```python
from build123d import *

# Parameters (mm, degrees)
SKETCH2_R           = 25.4
BASE_CYLINDER_DEPTH = 19.05
SKETCH3_R           = 56.35625
AFT_FLANGE_DEPTH    = 9.525
BOLT_CIRCLE_D       = 2.8702
BOLT_CIRCLE_DEPTH   = 9.525


with BuildPart() as part:
    # Sketch2 → Base Cylinder (new body)
    with BuildSketch(Plane(origin=(0, 0, 0), x_dir=(1, 0, 0), z_dir=(0, 1, 0))):
        Circle(SKETCH2_R)
    extrude(amount=BASE_CYLINDER_DEPTH)

    # Sketch3 → Aft Flange (add)
    with BuildSketch(Plane.XZ):
        Circle(SKETCH3_R)
    extrude(amount=-AFT_FLANGE_DEPTH)

    # Bolt Circle
    with Locations(Plane(origin=(0, 0, 0), x_dir=(-1, 0, 0), z_dir=(0, -1, 0))):
        with Locations((-25.81275, -44.708994483), (-44.708994483, -25.81275), (-51.6255, 0), (-44.708994483, 25.81275), (-25.81275, 44.708994483), (0, 51.6255), (25.81275, 44.708994483), (44.708994483, 25.81275), (51.6255, 0), (44.708994483, -25.81275), (25.81275, -44.708994483), (0, -51.6255)):
            Hole(BOLT_CIRCLE_D / 2, depth=BOLT_CIRCLE_DEPTH)

    # Sketch17 → 3/8 NPT Tapped Hole1 (revolve, cut)
    with BuildSketch(Plane(origin=(0, 19.05, 0), x_dir=(0, 0, 1), z_dir=(1, 0, 0))):
        Polygon((0, 0), (0, 21.814582582), (7.1374, 17.526), (7.1374, 10.414), (8.263205494, 10.414), (8.5750146, 0), align=None)
    revolve(axis=Axis((0, 25.4, 0), (0, -1, 0)), mode=Mode.SUBTRACT)


solid = part.part
```
Check sheet for the modelled part. Datum: model origin and axes. Units: mm. A direction names the side the tool comes from. Coordinates: 2 decimals unless noted, no trailing zeros. Order: outer loops, then holes, each group sorted by start corner. A loop starts at its lowest first (then second) coordinate and runs counter-clockwise, first axis right, second up. Notation, with made-up numbers: (34.5, 6) -> (50.5, 6) arc R14 cw to (50.5, 19) -> close; hole circle Ø6 at (49.5, 58.5). An arc over 180 degrees is marked (long way). Write item = value, one per line. Start each with the question number.
1) Cross-section at B-B (x = 16). Enter the section's corners in (y, z) (3 decimals).
2) Cross-section at D-D (z = 15.5). Enter the section's corners in (x, y) (3 decimals), then the cut area to 3 significant figures.
3) Cross-section at C-C (x = 0). Enter the section's corners in (y, z) (3 decimals), then the cut area to 3 significant figures.
4) Material ranges on L1, parallel to Z at x = 0, y = 5; L2, parallel to Z at x = -26.5, y = 2.5; L3, parallel to Y at x = 25.5, z = 16 (3 decimals), recorded low to high.
5) Access from +Z, -Z, +X, -X, +Y, -Y to the whole of each face (thin tool, end or side, straight path). Record for faces 4 (the cylindrical face through (-5.506, 14.221, 24.796)), 5 (the cylindrical face through (-46.143, 4.829, -25.876)).
6) Mould release check, pull along X, two halves, no side actions. Record for faces 1 (the cylindrical face through (-25.15, 4.83, 45.98)), 2 (the cylindrical face through (-56.3, 4.7, 2.5)), 3 (the flat face through (24, 9.525, -12)): +X half, -X half, draft (parallel to the pull), parting line (faces both ways), or undercut.
7) Cross-section at A-A (z = 0). Enter the section's corners in (x, y) (3 decimals).
8) Go/stop test with flat-tipped pins: P1, Ø2.5, axis at x = 25.81, z = 44.71, coming from the -Y side; P2, Ø3.5, axis at x = 44.71, z = 25.81, coming from the -Y side; P3, Ø6, axis at y = 6, z = 38.5, coming from the +X side; P4, Ø3.5, axis at x = 51.63, z = 0, coming from the +Y side (3 decimals). Record where each tip stops, or that it passes through.
Ans:
q1.outline = (0, -54.037) -> (9.525, -54.037) -> (9.525, -19.727) -> (19.05, -19.727) -> (19.05, 19.727) -> (9.525, 19.727) -> (9.525, 54.037) -> (0, 54.037) -> close
q2.outline = (-54.183, 0) -> (54.183, 0) -> (54.183, 9.525) -> (20.122, 9.525) -> (20.122, 19.05) -> (-20.122, 19.05) -> (-20.122, 9.525) -> (-54.183, 9.525) -> close
q2.area = 1,420 mm²
q3.outline = (0, -56.356) -> (9.525, -56.356) -> (9.525, -53.061) -> (0, -53.061) -> close; (0, -50.19) -> (9.525, -50.19) -> (9.525, -25.4) -> (19.05, -25.4) -> (19.05, -8.575) -> (8.636, -8.263) -> (8.636, -7.137) -> (1.524, -7.137) -> (0, -4.601) -> close; (0, 4.601) -> (1.524, 7.137) -> (8.636, 7.137) -> (8.636, 8.263) -> (19.05, 8.575) -> (19.05, 25.4) -> (9.525, 25.4) -> (9.525, 50.19) -> (0, 50.19) -> close; (0, 53.061) -> (9.525, 53.061) -> (9.525, 56.356) -> (0, 56.356) -> close
q3.area = 1,210 mm²
q4.L1 = -56.36 to -53.06, -50.19 to -7.14, 7.14 to 50.19, 53.06 to 56.36
q4.L2 = -49.74 to -45.97, -43.45 to 43.45, 45.97 to 49.74
q4.L3 = 0 to 9.525
q5.face_4 = +Y
q5.face_5 = +Y, -Y
q6.face_1 = undercut
q6.face_2 = parting line
q6.face_3 = draft
q7.outline = (-56.356, 0) -> (-53.061, 0) -> (-53.061, 9.525) -> (-56.356, 9.525) -> close; (-50.19, 0) -> (-4.601, 0) -> (-7.137, 1.524) -> (-7.137, 8.636) -> (-8.263, 8.636) -> (-8.575, 19.05) -> (-25.4, 19.05) -> (-25.4, 9.525) -> (-50.19, 9.525) -> close; (4.601, 0) -> (50.19, 0) -> (50.19, 9.525) -> (25.4, 9.525) -> (25.4, 19.05) -> (8.575, 19.05) -> (8.263, 8.636) -> (7.137, 8.636) -> (7.137, 1.524) -> close; (53.061, 0) -> (56.356, 0) -> (56.356, 9.525) -> (53.061, 9.525) -> close
q8.P1 = through
q8.P2 = 0
q8.P3 = 43.77
q8.P4 = 9.525
